from build123d import *

# Parameters (mm, degrees)
SKETCH1_W                = 20
SKETCH1_H                = 30
BOSS_EXTRUDE1_DEPTH      = 3
M3_CLEARANCE_HOLE1_D     = 3.2
M3_CLEARANCE_HOLE1_DEPTH = 5
M3_CLEARANCE_HOLE1_TIP   = 0.96137699
SKETCH4_R                = 4.875
CUT_EXTRUDE1_DEPTH       = 3
BOSS_EXTRUDE2_START      = 20
SKETCH5_R                = 5.5
SKETCH5_R_2              = 4.875
BOSS_EXTRUDE2_DEPTH      = 20


with BuildPart() as part:
    # Sketch1 → Boss-Extrude1 (new body)
    with BuildSketch(Plane(origin=(0, 0, 0), x_dir=(1, 0, 0), z_dir=(0, 1, 0))):
        Rectangle(SKETCH1_W, SKETCH1_H)
    extrude(amount=BOSS_EXTRUDE1_DEPTH)

    # M3 Clearance Hole1
    with Locations(Plane(origin=(-7.5, 3, 11), x_dir=(0, 0, 1), z_dir=(0, 1, 0))):
        with Locations((0, 0), (0, 15)):
            Hole(M3_CLEARANCE_HOLE1_D / 2, depth=M3_CLEARANCE_HOLE1_DEPTH)
            with Locations((0, 0, -(M3_CLEARANCE_HOLE1_DEPTH + M3_CLEARANCE_HOLE1_TIP / 2))):  # 118° drill point
                Cone(0, M3_CLEARANCE_HOLE1_D / 2, M3_CLEARANCE_HOLE1_TIP, mode=Mode.SUBTRACT)

    # Sketch4 → Cut-Extrude1 (cut)
    with BuildSketch(Plane(origin=(0, 3, 0), x_dir=(1, 0, 0), z_dir=(0, 1, 0))):
        with Locations(Location((0, 5.95, 0), (0, 0, 270))):
            Circle(SKETCH4_R)
    extrude(amount=-CUT_EXTRUDE1_DEPTH, mode=Mode.SUBTRACT)

    # Sketch5 → Boss-Extrude2 (add)
    with BuildSketch(Plane(origin=(0, 3, 0), x_dir=(1, 0, 0), z_dir=(0, 1, 0)).offset(BOSS_EXTRUDE2_START)):
        with Locations(Location((0, 5.95, 0), (0, 0, 90))):
            Circle(SKETCH5_R)
        with Locations(Location((0, 5.95, 0), (0, 0, 270))):
            Circle(SKETCH5_R_2, mode=Mode.SUBTRACT)
    extrude(amount=-BOSS_EXTRUDE2_DEPTH)


solid = part.part
Source: CAD feature listing. Evaluate the final solid. Frame: model axes, mm. Give positions to 0.01 mm unless a question says otherwise; leave off trailing zeros. Write each loop counter-clockwise with the first axis right and the second up, starting at its lowest first coordinate (ties: lowest second). Pieces come first, ordered by that corner, then holes. Notation, with made-up numbers: (54, -29.75) -> (63, -29.75) arc R25 ccw to (63, 0.25) -> close; hole circle Ø11 at (48, 20.5). An arc over 180 degrees is marked (long way). Return JSON: item names as keys, results as strings. Group by question number.
1. Section B-B, the plane z = -5.95. Output: boundary loops of the cut face in (x, y) (3 decimals), then the cut area to 4 significant figures.
2. Section D-D, the plane x = 0. Output: boundary loops of the cut face in (y, z) (3 decimals).
3. Pin query (flat end, axial travel): pin 1 Ø12 at (x, z) = (-6.5, -6) entering from -Y; pin 2 Ø1 at (y, z) = (11, -7) entering from +X; pin 3 Ø3 at (x, y) = (8, 13.5) entering from +Z; pin 4 Ø4 at (x, z) = (-7.5, 11) entering from +Y. Return the tip coordinate at first contact, or that it passes through.
4. Section C-C, the plane z = 11. Output: boundary loops of the cut face in (x, y).
5. Material intervals for line 1 (X direction, y = 0.6, z = 11); line 2 (X direction, y = 16.5, z = -5.95) (3 decimals); line 3 (X direction, y = 12, z = -4.5), sorted ascending. Write a range as from..to.
6. Section A-A, the plane x = 7.5. Output: boundary loops of the cut face in (y, z).
7. Mould query, pull axis Z, two halves, no side actions, for faces 1 (the face through (0, 1, 15)), 2 (the face through (5, 23, -5)), 3 (the face through (1.46, 11.66, -1.3)), 4 (the face through (2.11, 13.14, -11.03)). Classes: +Z half, -Z half, draft (parallel to the pull), parting line (faces both ways), or undercut.
Determined:
{
 "1": {"outline": "(-10, 0) -> (-4.875, 0) -> (-4.875, 23) -> (-5.5, 23) -> (-5.5, 3) -> (-10, 3) -> close; (4.875, 0) -> (10, 0) -> (10, 3) -> (5.5, 3) -> (5.5, 23) -> (4.875, 23) -> close", "area": "55.75 mm2"},
 "2": {"outline": "(0, -15) -> (3, -15) -> (3, -11.45) -> (23, -11.45) -> (23, -10.825) -> (0, -10.825) -> close; (0, -1.075) -> (23, -1.075) -> (23, -0.45) -> (3, -0.45) -> (3, 15) -> (0, 15) -> close"},
 "3": {"pin 1": "stops at y = 0", "pin 2": "stops at x = 5.47", "pin 3": "passes through", "pin 4": "stops at y = 3"},
 "4": {"outline": "(-10, 0) -> (-9.1, 0) -> (-9.1, 3) -> (-10, 3) -> close; (-5.9, 0) -> (5.9, 0) -> (5.9, 3) -> (-5.9, 3) -> close; (9.1, 0) -> (10, 0) -> (10, 3) -> (9.1, 3) -> close"},
 "5": {"line 1": "x = -10..-9.1, -5.9..5.9, 9.1..10", "line 2": "x = -5.5..-4.875, 4.875..5.5", "line 3": "x = -5.31..-4.65, 4.65..5.31"},
 "6": {"outline": "(0, -15) -> (3, -15) -> (3, 9.4) -> (0, 9.4) -> close; (0, 12.6) -> (3, 12.6) -> (3, 15) -> (0, 15) -> close"},
 "7": {"face 1": "+Z half", "face 2": "draft", "face 3": "undercut", "face 4": "parting line"}
}
